from build123d import *

# Parameters (mm, degrees)
F0_W     = 45
F0_H     = 45
F1_DEPTH = 100
F2_R     = 5
F3_R     = 10
F4_DEPTH = 45
F5_R     = 12.5
F6_DEPTH = 45


with BuildPart() as f1:
    # F0 (on Front) → F1 (new body)
    with BuildSketch(Plane.XZ):
        with Locations((-22.5, 22.5)):
            Rectangle(F0_W, F0_H)
    extrude(amount=F1_DEPTH)

    # F2
    f2_edges = [f1.edges().sort_by_distance(p)[0] for p in [
        (-22.5, -100, 0),
        (0, -100, 22.5),
        (-22.5, -100, 45),
        (-45, -100, 22.5),
        (-45, -50, 45),
        (-45, -50, 0),
        (-45, 0, 22.5),
        (0, -50, 45),
        (-22.5, 0, 45),
        (0, -50, 0),
        (0, 0, 22.5),
        (-22.5, 0, 0),
    ]]
    fillet(f2_edges, radius=F2_R)

    # F3 (on face) → F4 (cut)
    with BuildSketch(Plane.XY.offset(45)):
        with Locations((-22.5, -77.5)):
            Circle(F3_R)
    extrude(amount=-F4_DEPTH, mode=Mode.SUBTRACT)

    # F5 (on face) → F6 (cut)
    with BuildSketch(Plane(origin=(-45, 0, 0), x_dir=(0, -1, 0), z_dir=(-1, 0, 0))):
        with Locations((22.5, 22.5)):
            Circle(F5_R)
    extrude(amount=-F6_DEPTH, mode=Mode.SUBTRACT)


solid = f1.part
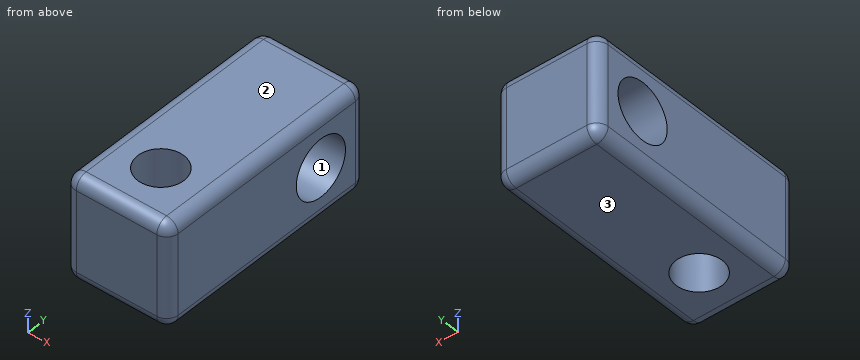
Here's how the part is built. I have some questions about the finished solid (model axes, mm). Face numbers are marked on the shaded views. Coordinates: 2 decimals unless noted, no trailing zeros. Loops run counter-clockwise (first coordinate to the right, second up) from the corner with the lowest first, then second, coordinate; pieces in that order, holes last. Notation, with made-up numbers: (41, 17.5) -> (72, 17.5) arc R28 ccw to (72, 54.5) -> close; hole circle Ø6 at (25.5, 87.5). An arc over 180 degrees is marked (long way). Use one line per item in the form item = value. Start each with the question number.
(1) If we section it at B-B (z = 22.5): Please give me the cut outline in (x, y).
(2) If we section it at A-A (x = -22.5): Please give me the cut outline in (y, z).
(3) We'd pull the mould along Z, two halves only. Please class the marked faces 1, 2 and 3: pulls with the +Z half, pulls with the -Z half, needs draft (parallel to the pull), parting line crosses it, or undercut.
(4) If we section it at D-D (x = -38.5): Please give me the cut outline in (y, z), then the cut area to 3 significant figures.
(5) Please list where these lines run through material, in increasing order: line 1 along Y through (x, z) = (-22, 23); line 2 along Y through (x, z) = (-22, 17); line 3 along Z through (x, y) = (-23.5, -22.5).
(6) If we section it at C-C (y = -77.5): Please give me the cut outline in (x, z).
Verdict:
q1.outline = (-45, -95) arc R5 ccw to (-40, -100) -> (-5, -100) arc R5 ccw to (0, -95) -> (0, -35) -> (-45, -35) -> close; (-45, -10) -> (0, -10) -> (0, -5) arc R5 ccw to (-5, 0) -> (-40, 0) arc R5 ccw to (-45, -5) -> close; hole circle Ø20 at (-22.5, -77.5)
q2.outline = (-100, 5) arc R5 ccw to (-95, 0) -> (-87.5, 0) -> (-87.5, 45) -> (-95, 45) arc R5 ccw to (-100, 40) -> close; (-67.5, 0) -> (-5, 0) arc R5 ccw to (0, 5) -> (0, 40) arc R5 ccw to (-5, 45) -> (-67.5, 45) -> close; hole circle Ø25 at (-22.5, 22.5)
q3.face_1 = undercut
q3.face_2 = pulls with the +Z half
q3.face_3 = pulls with the -Z half
q4.outline = (-100, 5) arc R5 ccw to (-95, 0) -> (-5, 0) arc R5 ccw to (0, 5) -> (0, 40) arc R5 ccw to (-5, 45) -> (-95, 45) arc R5 ccw to (-100, 40) -> close; hole circle Ø25 at (-22.5, 22.5)
q4.area = 3,990 mm²
q5.line_1 = -100 to -87.49, -67.51 to -34.99, -10.01 to 0
q5.line_2 = -100 to -87.49, -67.51 to -33.72, -11.28 to 0
q5.line_3 = 0 to 10, 35 to 45
q6.outline = (-45, 5) arc R5 ccw to (-40, 0) -> (-32.5, 0) -> (-32.5, 45) -> (-40, 45) arc R5 ccw to (-45, 40) -> close; (-12.5, 0) -> (-5, 0) arc R5 ccw to (0, 5) -> (0, 40) arc R5 ccw to (-5, 45) -> (-12.5, 45) -> close
